Build history of the part. All positions in model axes, mm. Face numbers are marked on the shaded views. A direction names the side the tool comes from. Round coordinates to 2 decimals unless told otherwise and drop trailing zeros. Write each loop counter-clockwise with the first axis right and the second up, starting at its lowest first coordinate (ties: lowest second). Pieces come first, ordered by that corner, then holes. Notation, with made-up numbers: (30, 70) - (65, 70) arc R24 cw to (65, 97) - close; hole circle Ø8 at (-4.75, -8). An arc over 180 degrees is marked (long way). One line per question, with ' | ' between items.
from build123d import *

# Parameters (mm, degrees)
BOSS_EXTRUDE1_DEPTH = 40
FILLET1_R           = 10
SKETCH3_R           = 7.989564155
SKETCH3_R_2         = 5.892903955
SKETCH3_R_3         = 5.960312231
SKETCH3_R_4         = 6.003710983
SKETCH3_R_5         = 5.972502613
BOSS_EXTRUDE2_DEPTH = 5


with BuildPart() as part:
    # Sketch2 → Boss-Extrude1 (new body)
    with BuildSketch(Plane.XY):
        Polygon((10.161880784, 60.526315789), (60.161880784, 60.526315789), (92.220072964, 99.539400074), (124.278265144, 60.526315789), (174.278265144, 60.526315789), (124.413003502, 27.157832435), (152.220072964, -14.396552267), (92.220072964, 6.015037594), (32.220072964, -14.396552267), (60.027142426, 27.157832435), align=None)
    extrude(amount=BOSS_EXTRUDE1_DEPTH)

    # Fillet1
    fillet1_edges = [part.edges().sort_by_distance(p)[0] for p in [
        (10.161880784, 60.526315789, 20),
        (92.220072964, 99.539400074, 20),
        (174.278265144, 60.526315789, 20),
        (124.413003502, 27.157832435, 20),
        (152.220072964, -14.396552267, 20),
        (92.220072964, 6.015037594, 20),
        (32.220072964, -14.396552267, 20),
        (60.027142426, 27.157832435, 20),
    ]]
    fillet(fillet1_edges, radius=FILLET1_R)

    # Sketch3 → Boss-Extrude2 (add)
    with BuildSketch(Plane.XY.offset(40)):
        with Locations((92.220072964, 72.831646457)):
            Circle(SKETCH3_R)
        with Locations((43.086739991, 50.526315789)):
            Circle(SKETCH3_R_2)
        with Locations((56.950737692, 4.579469525)):
            Circle(SKETCH3_R_3)
        with Locations((127.489408235, 4.579469525)):
            Circle(SKETCH3_R_4)
        with Locations((141.353405936, 50.526315789)):
            Circle(SKETCH3_R_5)
    extrude(amount=BOSS_EXTRUDE2_DEPTH)


solid = part.part
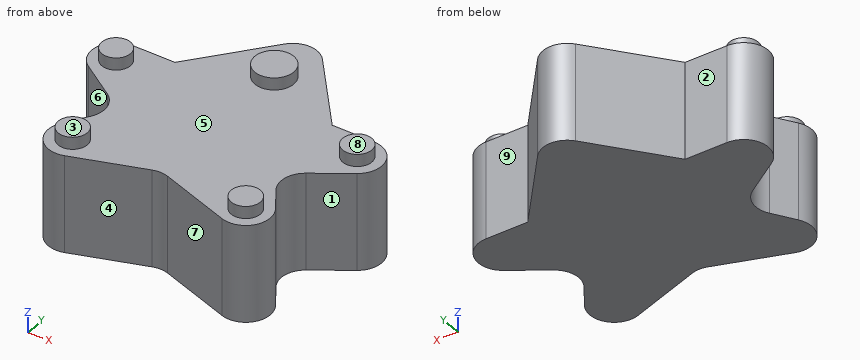
Q1. Drop flat-ended pins along their axis: pin 1 (2 mm diameter, centred on y = 57, z = 25.5, fed in from +X); pin 2 (5 mm diameter, centred on x = 52, z = 14, fed in from +Y); pin 3 (12 mm diameter, centred on y = 13.5, z = 40, fed in from +X). Give the stop position or say it passes through.
Found:
pin 1: x = 149.72 | pin 2: y = 60.53 | pin 3: x = 137.05
Q2. Saw through at A-A, the plane z = 35.5. List the corners of the cut face in (x, y), then the cut area to 3 significant figures.
Found:
outline: (37.53, 42.22) - (51.72, 32.72) arc R10 cw to (54.47, 18.85) - (48.64, 10.14) arc R10 ccw to (60.17, -4.89) - (89, 4.92) arc R10 cw to (95.44, 4.92) - (124.27, -4.89) arc R10 ccw to (135.8, 10.14) - (129.97, 18.85) arc R10 cw to (132.72, 32.72) - (146.91, 42.22) arc R10 ccw to (141.35, 60.53) - (124.28, 60.53) - (99.95, 90.14) arc R10 ccw to (84.49, 90.14) - (60.16, 60.53) - (43.09, 60.53) arc R10 ccw to start | area: 6,940 mm^2
Q3. Pull direction Y, two halves, no side cores. Call the marked faces 1, 2, 3 and 4: +Y half, -Y half, draft (parallel to the pull), parting line (faces both ways), or undercut.
Found:
face 1: undercut | face 2: +Y half | face 3: draft | face 4: -Y half
Q4. Drill centre lines: L1, parallel to X at y = 24, z = 10; L2, parallel to Z at x = 123.5, y = 16; L3, parallel to Y at x = 50.5, z = 21. Where is each one in solid material? Low to high. Write a range as from..to.
Found:
L1: 56.15..128.29 | L2: 0..40 | L3: -3.06..12.92, 33.53..60.53
Q5. Which spindle directions (+Z, -Z, +X, -X, +Y, -Y) get a long thin tool onto all of the face, cutting with end or side? Do the marked faces 5, 6, 7, 8 and 9. Say none if no direction does.
Found:
face 5: +Z | face 6: +Z, -Z, -X | face 7: +Z, -Z, -Y | face 8: +Z, +X, -X, +Y, -Y | face 9: +Z, -Z, +X, +Y
Q6. Saw through at D-D, the plane y = 35.5. List the corners of the cut face in (x, z), then the cut area to 3 significant figures.
Found:
outline: (47.56, 0) - (136.88, 0) - (136.88, 40) - (47.56, 40) - close | area: 3,570 mm^2
Q7. Saw through at C-C, the plane x = 82. List the corners of the cut face in (y, z), then the cut area to 3 significant figures.
Found:
outline: (2.54, 0) - (87.1, 0) - (87.1, 40) - (2.54, 40) - close | area: 3,380 mm^2
Q8. Saw through at B-B, the plane y = 48. List the corners of the cut face in (x, z), then the cut area to 3 significant figures.
Found:
outline: (33.41, 0) - (151.03, 0) - (151.03, 40) - (146.77, 40) - (146.77, 45) - (135.94, 45) - (135.94, 40) - (48.41, 40) - (48.41, 45) - (37.76, 45) - (37.76, 40) - (33.41, 40) - close | area: 4,810 mm^2
